from build123d import *

# Parameters (mm, degrees)
CROQUIS1_R              = 1.5
CROQUIS1_W              = 21.7
CROQUIS1_H              = 10.8
SALIENTE_EXTRUIR1_DEPTH = 3
CORTAR_EXTRUIR2_DEPTH   = 3
REDONDEO1_R             = 1
REDONDEO2_R             = 0.25


with BuildPart() as part:
    # Croquis1 → Saliente-Extruir1 (new body)
    with BuildSketch(Plane.XY):
        with BuildLine():
            Line((-50, 25), (-50, -25))
            ThreePointArc((-50, -25), (-49.267766953, -26.767766953), (-47.5, -27.5))
            Line((-47.5, -27.5), (-37.9, -27.5))
            Line((-37.9, -27.5), (-37.9, -30.5))
            Line((-37.9, -30.5), (-27.9, -30.5))
            Line((-27.9, -30.5), (-27.9, -33.6))
            Line((-27.9, -33.6), (-37.9, -33.6))
            Line((-37.9, -33.6), (-37.9, -35.6))
            Line((-37.9, -35.6), (-25.4, -35.6))
            ThreePointArc((-25.4, -35.6), (-23.632233047, -34.867766953), (-22.9, -33.1))
            Line((-22.9, -33.1), (-22.9, -27.5))
            Line((-22.9, -27.5), (22.9, -27.5))
            Line((22.9, -27.5), (22.9, -33.1))
            ThreePointArc((22.9, -33.1), (23.632233047, -34.867766953), (25.4, -35.6))
            Line((25.4, -35.6), (37.9, -35.6))
            Line((37.9, -35.6), (37.9, -33.6))
            Line((37.9, -33.6), (27.9, -33.6))
            Line((27.9, -33.6), (27.9, -30.5))
            Line((27.9, -30.5), (37.9, -30.5))
            Line((37.9, -30.5), (37.9, -27.5))
            Line((37.9, -27.5), (47.5, -27.5))
            ThreePointArc((47.5, -27.5), (49.267766953, -26.767766953), (50, -25))
            Line((50, -25), (50, 25))
            ThreePointArc((50, 25), (49.267766953, 26.767766953), (47.5, 27.5))
            Line((47.5, 27.5), (37.9, 27.5))
            Line((37.9, 27.5), (37.9, 30.5))
            Line((37.9, 30.5), (27.9, 30.5))
            Line((27.9, 30.5), (27.9, 33.6))
            Line((27.9, 33.6), (37.9, 33.6))
            Line((37.9, 33.6), (37.9, 35.6))
            Line((37.9, 35.6), (25.4, 35.6))
            ThreePointArc((25.4, 35.6), (23.632233047, 34.867766953), (22.9, 33.1))
            Line((22.9, 33.1), (22.9, 27.5))
            Line((22.9, 27.5), (-22.9, 27.5))
            Line((-22.9, 27.5), (-22.9, 33.1))
            ThreePointArc((-22.9, 33.1), (-23.632233047, 34.867766953), (-25.4, 35.6))
            Line((-25.4, 35.6), (-37.9, 35.6))
            Line((-37.9, 35.6), (-37.9, 33.6))
            Line((-37.9, 33.6), (-27.9, 33.6))
            Line((-27.9, 33.6), (-27.9, 30.5))
            Line((-27.9, 30.5), (-37.9, 30.5))
            Line((-37.9, 30.5), (-37.9, 27.5))
            Line((-37.9, 27.5), (-47.5, 27.5))
            ThreePointArc((-47.5, 27.5), (-49.267766953, 26.767766953), (-50, 25))
        make_face()
        with Locations((-14, 17.663397979)):
            Circle(CROQUIS1_R, mode=Mode.SUBTRACT)
        with Locations(Location((14, 17.663397979, 0), (0, 0, 180))):
            Circle(CROQUIS1_R, mode=Mode.SUBTRACT)
        with Locations((14, 3.643397979)):
            Circle(CROQUIS1_R, mode=Mode.SUBTRACT)
        with Locations(Location((-14, 3.643397979, 0), (0, 0, 180))):
            Circle(CROQUIS1_R, mode=Mode.SUBTRACT)
        with Locations((0, 10.653397979)):
            Rectangle(CROQUIS1_W, CROQUIS1_H, mode=Mode.SUBTRACT)
    extrude(amount=SALIENTE_EXTRUIR1_DEPTH)

    # Croquis2 → Cortar-Extruir2 (cut, symmetric)
    with BuildSketch(Plane.XY):
        with BuildLine():
            Line((-17.5, -17.5), (17.5, -17.5))
            ThreePointArc((17.5, -17.5), (19.267766953, -18.232233047), (20, -20))
            Line((20, -20), (20, -37.5))
            Line((20, -37.5), (-20, -37.5))
            Line((-20, -37.5), (-20, -20))
            ThreePointArc((-20, -20), (-19.267766953, -18.232233047), (-17.5, -17.5))
        make_face()
    extrude(amount=CORTAR_EXTRUIR2_DEPTH, both=True, mode=Mode.SUBTRACT)

    # Redondeo1
    redondeo1_edges = [part.edges().sort_by_distance(p)[0] for p in [
        (10.85, 5.253397979, 1.5),
        (10.85, 16.053397979, 1.5),
        (-10.85, 16.053397979, 1.5),
        (-10.85, 5.253397979, 1.5),
        (20, -27.5, 1.5),
        (-20, -27.5, 1.5),
        (-37.9, 27.5, 1.5),
        (-37.9, 35.6, 1.5),
        (-22.9, 27.5, 1.5),
        (22.9, 27.5, 1.5),
        (37.9, 35.6, 1.5),
        (37.9, 27.5, 1.5),
        (37.9, -27.5, 1.5),
        (37.9, -35.6, 1.5),
        (22.9, -27.5, 1.5),
        (-22.9, -27.5, 1.5),
        (-37.9, -35.6, 1.5),
        (-37.9, -27.5, 1.5),
    ]]
    fillet(redondeo1_edges, radius=REDONDEO1_R)

    # Redondeo2
    redondeo2_edges = [part.edges().sort_by_distance(p)[0] for p in [
        (-37.9, 30.5, 1.5),
        (-27.9, 30.5, 1.5),
        (-27.9, 33.6, 1.5),
        (-37.9, 33.6, 1.5),
        (37.9, 33.6, 1.5),
        (27.9, 33.6, 1.5),
        (27.9, 30.5, 1.5),
        (37.9, 30.5, 1.5),
        (37.9, -30.5, 1.5),
        (27.9, -30.5, 1.5),
        (27.9, -33.6, 1.5),
        (37.9, -33.6, 1.5),
        (-37.9, -33.6, 1.5),
        (-27.9, -33.6, 1.5),
        (-27.9, -30.5, 1.5),
        (-37.9, -30.5, 1.5),
    ]]
    fillet(redondeo2_edges, radius=REDONDEO2_R)


solid = part.part
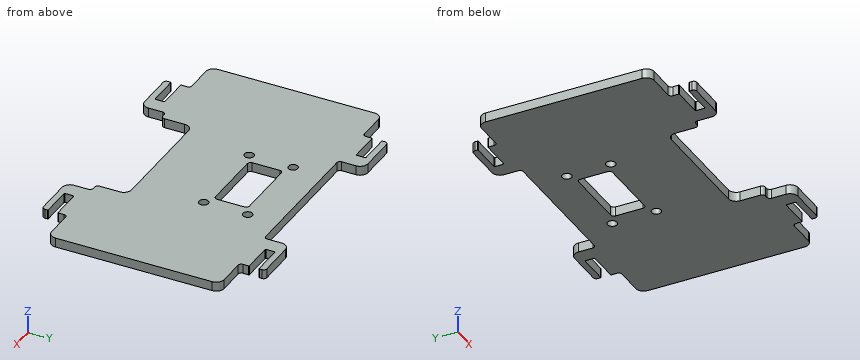
Design review of the part built by this model. Coordinates are the model's own, in mm. Round coordinates to 2 decimals unless told otherwise and drop trailing zeros. Write each loop counter-clockwise with the first axis right and the second up, starting at its lowest first coordinate (ties: lowest second). Pieces come first, ordered by that corner, then holes. Notation, with made-up numbers: M -9,62 L 20,62 A20 ccw 20,84 Z; hole C 61.25,-24.75 d5. An arc over 180 degrees is marked long. One line per item, written item: value. Start each with the question number.
1. Take a section at A-A on x = -1.5. State the section outline as (y, z) points, then the cut area to 3 significant figures.
2. Take a section at C-C on x = -41. State the section outline as (y, z) points.
3. Take a section at B-B on x = 14. State the section outline as (y, z) points.
4. Take a section at D-D on z = 0.85. State how many separate pieces and enclosed holes the cut face has, then the cut area to 3 significant figures.
5. To check wall thickness, follow probe 1 along Y at (x, z) = (-14, 1.35); probe 2 along X at (y, z) = (31.5, 0.2); probe 3 along X at (y, z) = (14, 0.9). State the ranges of each line that lie inside material, in increasing order. Write a range as from..to.
6. Clearance check with flat-ended pins moving along their axes: P1, Ø1.4, axis at y = 29.5, z = 2, coming from the -X side; P2, Ø0.9, axis at y = -29.5, z = 1.5, coming from the +X side; P3, Ø1.3, axis at y = -32.5, z = 1.5, coming from the -X side. State where each tip first meets the part, or that it passes through.
Computed:
1. outline: M -17.5,0 L 5.25,0 L 5.25,3 L -17.5,3 Z; M 16.05,0 L 27.5,0 L 27.5,3 L 16.05,3 Z
1. area: 103 mm²
2. outline: M -27.5,0 L 27.5,0 L 27.5,3 L -27.5,3 Z
3. outline: M -17.5,0 L 2.14,0 L 2.14,3 L -17.5,3 Z; M 5.14,0 L 16.16,0 L 16.16,3 L 5.14,3 Z; M 19.16,0 L 27.5,0 L 27.5,3 L 19.16,3 Z
4. separate pieces: 1
4. enclosed holes: 5
4. area: 5,190 mm²
5. probe 1: y = -17.5..2.14, 5.14..16.16, 19.16..27.5
5. probe 2: x = -27.9..-22.9, 22.9..27.9
5. probe 3: x = -50..-10.85, 10.85..50
6. P1: stops at x = -37.9
6. P2: stops at x = 37.9
6. P3: stops at x = -27.9
